```python
from build123d import *

# Parameters (mm, degrees)
BOSS_EXTRUDE1_DEPTH      = 8
SKETCH3_R                = 4
CUT_EXTRUDE1_DEPTH       = 59.516173282
SKETCH4_R                = 6.51
CUT_EXTRUDE2_DEPTH       = 5
SKETCH12_R               = 9
BOSS_EXTRUDE2_DEPTH      = 8
SKETCH13_R               = 2.015
CUT_EXTRUDE8_DEPTH       = 59.516173282
CUT_EXTRUDE10_DEPTH      = 58.40115448
CUT_EXTRUDE10_DEPTH_BACK = 58.40115448
SKETCH14_R               = 1.51


with BuildPart() as part:
    # Sketch1 → Boss-Extrude1 (new body)
    with BuildSketch(Plane.XY):
        with BuildLine():
            Line((0, 0), (40, 0))
            ThreePointArc((40, 0), (56.123903424, 5.5), (40, 11))
            Line((40, 11), (0, 11))
            Line((0, 11), (0, 0))
        make_face()
    extrude(amount=BOSS_EXTRUDE1_DEPTH)

    # Sketch3 → Cut-Extrude1 (cut, through all)
    with BuildSketch(Plane.XY.offset(8)):
        with Locations((47.123903424, 5.5)):
            Circle(SKETCH3_R)
    extrude(amount=-CUT_EXTRUDE1_DEPTH, mode=Mode.SUBTRACT)

    # Sketch4 → Cut-Extrude2 (cut)
    with BuildSketch(Plane.XY.offset(8)):
        with Locations((47.123903424, 5.5)):
            Circle(SKETCH4_R)
    extrude(amount=-CUT_EXTRUDE2_DEPTH, mode=Mode.SUBTRACT)

    # Sketch12 → Boss-Extrude2 (add)
    with BuildSketch(Plane.XY.offset(8)):
        with Locations((-2.876096576, 5.5)):
            Circle(SKETCH12_R)
    extrude(amount=-BOSS_EXTRUDE2_DEPTH)

    # Sketch13 → Cut-Extrude8 (cut, through all)
    with BuildSketch(Plane.XY.offset(8)):
        with Locations((-2.876096576, 5.5)):
            Circle(SKETCH13_R)
    extrude(amount=-CUT_EXTRUDE8_DEPTH, mode=Mode.SUBTRACT)

    # Sketch14 → Cut-Extrude10 (cut, two sides: drawn at the far end of the back side and taken through both)
    with BuildSketch(Plane(origin=(0, 5.5, 0), x_dir=(1, 0, 0), z_dir=(0, 1, 0)).offset(-CUT_EXTRUDE10_DEPTH_BACK)):
        with Locations(Location((-2.876096576, -4, 0), (0, 0, 270))):
            Circle(SKETCH14_R)
    extrude(amount=CUT_EXTRUDE10_DEPTH + CUT_EXTRUDE10_DEPTH_BACK, mode=Mode.SUBTRACT)


solid = part.part
```
Here's how the part is built. I have some questions about the finished solid (model axes, mm). A direction names the side the tool comes from. Give positions to 0.01 mm unless a question says otherwise; leave off trailing zeros. Write each loop counter-clockwise with the first axis right and the second up, starting at its lowest first coordinate (ties: lowest second). Pieces come first, ordered by that corner, then holes. Notation, with made-up numbers: M -13,31.25 L 7,31.25 A23 cw 7,49.25 Z; hole C -35.75,0.25 d2. An arc over 180 degrees is marked long. Put each result on its own line as item: value. Start each with the question number.
Item 1: If we section it at B-B, the plane z = 4: Write out the boundary of the cut face in (x, y) (3 decimals), then the cut area to 3 significant figures.
Item 2: On a 3-axis mill with a long thin cutter (end or side, diameter ignored), from which of +Z, -Z, +X, -X, +Y, -Y can I reach the whole of each face in a straight line? I mean faces 1 (the flat face through (22, 6, 0)), 2 (the cylindrical face through (40.62, 5.79, 5.54)), 3 (the cylindrical face through (-4.89, 5.59, 4.06)), 4 (the flat face through (22, 11, 4)), 5 (the flat face through (22, 0, 4)). Say none if no direction works.
Item 3: I need wall thicknesses on L1, parallel to Z at x = -3, y = 9.25; L2, parallel to X at y = 13.5, z = 3.75; L3, parallel to X at y = -2, z = 4. Which ranges of each line are inside material? Lowest first, please. Write a range as from..to.
Item 4: Thinking about a two-plate mould opening in Y: for faces 6 (the cylindrical face through (-11.87, 5.81, 4.06)), 7 (the flat face through (14, 6, 8)), 8 (the cylindrical face through (50.82, 3.97, 1.52)), which applies, +Y half, -Y half, draft (parallel to the pull), parting line (faces both ways), or undercut?
Item 5: Will these pins go through, and if not, where does the flat tip stop? pin 1 (3 mm diameter, centred on y = 12.5, z = 1, fed in from +X); pin 2 (6.5 mm diameter, centred on x = 47, y = 8.5, fed in from +Z); pin 3 (6 mm diameter, centred on x = 25.5, y = 10, fed in from -Z); pin 4 (4 mm diameter, centred on x = 20, z = 3.5, fed in from +Y).
Item 6: If we section it at D-D, the plane x = 11.5: Write out the boundary of the cut face in (y, z), then the cut area to 3 significant figures.
Item 7: If we section it at C-C, the plane z = 7: Write out the boundary of the cut face in (x, y) (3 decimals), then the cut area to 3 significant figures.
Item 8: If we section it at A-A, the plane y = 5.5: Write out the boundary of the cut face in (x, z).
Values:
1. outline: M -4.386,-3.372 L -4.386,4.166 A2.015 cw -4.386,6.834 L -4.386,14.372 A9 ccw Z; M -1.366,-3.372 A9 ccw 4.248,0 L 40,0 A9 ccw long 40,11 L 4.248,11 A9 ccw -1.366,14.372 L -1.366,6.834 A2.015 cw -1.366,4.166 Z; hole C 47.124,5.5 d13.02
1. area: 685 mm²
2. face 1: -Z, +X, -X, +Y, -Y
2. face 2: +Z
2. face 3: +Z, -Z
2. face 4: +Z, -Z, +Y
2. face 5: +Z, -Z, -Y
3. L1: 0..2.5, 5.5..8
3. L2: -7..-4.37, -1.39..1.25, 43..51.25
3. L3: -7.85..-4.39, -1.37..2.1, 42.15..52.1
4. face 6: parting line
4. face 7: draft
4. face 8: undercut
5. pin 1: x = 54.25
5. pin 2: z = 3
5. pin 3: z = 0
5. pin 4: y = 11
6. outline: M 0,0 L 11,0 L 11,8 L 0,8 Z
6. area: 88.0 mm²
7. outline: M 4.248,0 L 40,0 A9 ccw long 40,11 L 4.248,11 A9 ccw long Z; hole C -2.876,5.5 d4.03; hole C 47.124,5.5 d13.02
7. area: 728 mm²
8. outline: M -11.88,0 L -4.89,0 L -4.89,8 L -11.88,8 Z; M -0.86,0 L 43.12,0 L 43.12,3 L 40.61,3 L 40.61,8 L -0.86,8 Z; M 51.12,0 L 56.12,0 L 56.12,8 L 53.63,8 L 53.63,3 L 51.12,3 Z
